Read the model definition and answer for the solid it produces. Units are mm, in the model's axes. A direction names the side the tool comes from. Round coordinates to 2 decimals unless told otherwise and drop trailing zeros. Order: outer loops, then holes, each group sorted by start corner. A loop starts at its lowest first (then second) coordinate and runs counter-clockwise, first axis right, second up. Notation, with made-up numbers: (-24.5, -32) -> (16.5, -32) arc R4 cw to (16.5, -27) -> close; hole circle Ø2 at (88, 30.25). An arc over 180 degrees is marked (long way). Use a Markdown table: item, result. Add a question column.
1. Section A-A, the plane z = 70 is taken. Give the vertices of the cut face in (x, y), then the cut area to 3 significant figures.
2. Given pin 1 (4 mm diameter, centred on x = -44.5, y = 31.5, fed in from +Z); pin 2 (1.5 mm diameter, centred on x = -26, y = 38, fed in from +Z); pin 3 (0.6 mm diameter, centred on x = 56, y = -38.5, fed in from +Z), each flat-ended and moving along its own axis, determine where each tip first touches the part or whether it passes through.
3. Consider L1, parallel to Y at x = -56, z = 75; L2, parallel to Z at x = 56.35, y = 33; L3, parallel to X at y = 22, z = 41.5. Determine where each line is inside the solid, lowest interval first. Write a range as [from, to].
4. Section D-D, the plane y = 16.5 is taken. Give the vertices of the cut face in (x, z).
5. The mould has two halves that part along X. Classify faces 1 (the face through (-57.5, -1, 38)), 2 (the face through (56.021, 32.805, 76.487)), 3 (the face through (-54.5, -1, 43)): +X half, -X half, draft (parallel to the pull), parting line (faces both ways), or undercut.
6. For faces 4 (the face through (-1, 37, 38)), 5 (the face through (-1, 39, 68)), 6 (the face through (56, 0, 72)), determine the directions among +Z, -Z, +X, -X, +Y, -Y from which every point of the face is accessible in a straight line to the end or side of a thin tool.
7. Section C-C, the plane x = -44 is taken. Give the vertices of the cut face in (y, z), then the cut area to 3 significant figures.
8. Section B-B, the plane z = 19 is taken. Give the vertices of the cut face in (x, y), then the cut area to 3 significant figures.
```python
from build123d import *

# Parameters (mm, degrees)
SKETCH1_W               = 80
SKETCH1_H               = 115
BOSS_EXTRUDE1_DEPTH     = 72
SKETCH3_W               = 109
SKETCH3_H               = 74
CUT_EXTRUDE1_DEPTH      = 1
CUT_EXTRUDE1_DEPTH_BACK = 65
SKETCH4_W               = 3
SKETCH4_H               = 6
BOSS_EXTRUDE2_DEPTH     = 6
SKETCH5_W               = 109
SKETCH5_H               = 3
CUT_EXTRUDE2_DEPTH      = 4
SKETCH6_R               = 1.5
CUT_EXTRUDE3_DEPTH      = 1
CUT_EXTRUDE3_DEPTH_BACK = 116
FILLET1_R               = 2
SKETCH7_R               = 0.5
CUT_EXTRUDE4_DEPTH      = 1
CUT_EXTRUDE4_DEPTH_BACK = 81


with BuildPart() as part:
    # Sketch1 → Boss-Extrude1 (new body)
    with BuildSketch(Plane(origin=(0, 0, 0), x_dir=(0, 1, 0), z_dir=(0, 0, 1))):
        Rectangle(SKETCH1_W, SKETCH1_H)
    extrude(amount=BOSS_EXTRUDE1_DEPTH)

    # Sketch3 → Cut-Extrude1 (cut, two sides)
    with BuildSketch(Plane.XY.offset(72)) as cut_extrude1_sk:
        Rectangle(SKETCH3_W, SKETCH3_H)
    extrude(amount=CUT_EXTRUDE1_DEPTH, mode=Mode.SUBTRACT)
    extrude(cut_extrude1_sk.sketch, amount=-CUT_EXTRUDE1_DEPTH_BACK, mode=Mode.SUBTRACT)

    # Sketch4 → Boss-Extrude2 (add)
    with BuildSketch(Plane.XY.offset(72)):
        with Locations((-56, 33)):
            Rectangle(SKETCH4_W, SKETCH4_H)
        with Locations((-56, -33)):
            Rectangle(SKETCH4_W, SKETCH4_H)
        with Locations((56, -33)):
            Rectangle(SKETCH4_W, SKETCH4_H)
        with Locations((56, 33)):
            Rectangle(SKETCH4_W, SKETCH4_H)
    extrude(amount=BOSS_EXTRUDE2_DEPTH)

    # Sketch5 → Cut-Extrude2 (cut)
    with BuildSketch(Plane.XY.offset(72)):
        with Locations((0, 38.5)):
            Rectangle(SKETCH5_W, SKETCH5_H)
        with Locations((0, -38.5)):
            Rectangle(SKETCH5_W, SKETCH5_H)
    extrude(amount=-CUT_EXTRUDE2_DEPTH, mode=Mode.SUBTRACT)

    # Sketch6 → Cut-Extrude3 (cut, two sides)
    with BuildSketch(Plane.YZ.offset(57.5)) as cut_extrude3_sk:
        with Locations((-33, 75)):
            Circle(SKETCH6_R)
        with Locations((33, 75)):
            Circle(SKETCH6_R)
    extrude(amount=CUT_EXTRUDE3_DEPTH, mode=Mode.SUBTRACT)
    extrude(cut_extrude3_sk.sketch, amount=-CUT_EXTRUDE3_DEPTH_BACK, mode=Mode.SUBTRACT)

    # Fillet1
    fillet1_edges = [part.edges().sort_by_distance(p)[0] for p in [
        (56, 30, 72),
        (56, 36, 72),
        (56, 30, 78),
        (56, 36, 78),
        (56, -36, 72),
        (56, -30, 72),
        (56, -36, 78),
        (56, -30, 78),
        (-56, -30, 72),
        (-56, -36, 72),
        (-56, -30, 78),
        (-56, -36, 78),
        (-56, 36, 72),
        (-56, 30, 72),
        (-56, 36, 78),
        (-56, 30, 78),
    ]]
    fillet(fillet1_edges, radius=FILLET1_R)

    # Sketch7 → Cut-Extrude4 (cut, two sides)
    with BuildSketch(Plane(origin=(0, 40, 0), x_dir=(-1, 0, 0), z_dir=(0, 1, 0))) as cut_extrude4_sk:
        with Locations((0, 34)):
            Circle(SKETCH7_R)
    extrude(amount=CUT_EXTRUDE4_DEPTH, mode=Mode.SUBTRACT)
    extrude(cut_extrude4_sk.sketch, amount=-CUT_EXTRUDE4_DEPTH_BACK, mode=Mode.SUBTRACT)


solid = part.part
```
Verdict:
| question | item | result |
|---|---|---|
| 1 | outline | (-57.5, -40) -> (-54.5, -40) -> (-54.5, 40) -> (-57.5, 40) -> close; (54.5, -40) -> (57.5, -40) -> (57.5, 40) -> (54.5, 40) -> close |
| 1 | area | 480 mm2 |
| 2 | pin 1 | stops at z = 7 |
| 2 | pin 2 | stops at z = 68 |
| 2 | pin 3 | stops at z = 72 |
| 3 | L1 | y = [-36, -34.5], [-31.5, -30], [30, 31.5], [34.5, 36] |
| 3 | L2 | z = [0, 73.5], [76.5, 78] |
| 3 | L3 | x = [-57.5, -54.5], [54.5, 57.5] |
| 4 | outline | (-57.5, 0) -> (57.5, 0) -> (57.5, 72) -> (54.5, 72) -> (54.5, 7) -> (-54.5, 7) -> (-54.5, 72) -> (-57.5, 72) -> close |
| 5 | face 1 | -X half |
| 5 | face 2 | draft |
| 5 | face 3 | undercut |
| 6 | face 4 | +Z |
| 6 | face 5 | +Z, +Y, -Y |
| 6 | face 6 | +Z, +X, -X |
| 7 | outline | (-40, 0) -> (40, 0) -> (40, 68) -> (37, 68) -> (37, 7) -> (-37, 7) -> (-37, 68) -> (-40, 68) -> close |
| 7 | area | 926 mm2 |
| 8 | outline | (-57.5, -40) -> (57.5, -40) -> (57.5, 40) -> (-57.5, 40) -> close; hole (-54.5, -37) -> (54.5, -37) -> (54.5, 37) -> (-54.5, 37) -> close |
| 8 | area | 1,130 mm2 |
